Here's how the part is built. I have some questions about the finished solid (model axes, mm). Face numbers are marked on the shaded views. Coordinates: 2 decimals unless noted, no trailing zeros. Write each loop counter-clockwise with the first axis right and the second up, starting at its lowest first coordinate (ties: lowest second). Pieces come first, ordered by that corner, then holes. Notation, with made-up numbers: (-37.75, -6) -> (4.25, -6) arc R12 ccw to (4.25, 5) -> close; hole circle Ø11 at (17, -13). An arc over 180 degrees is marked (long way). Put each result on its own line as item: value.
```python
from build123d import *

# Parameters (mm, degrees)
ESQUISSE1_R                  = 3.4
BOSS_EXTRU_1_DEPTH           = 28
ENL_V_MAT_EXTRU_1_DEPTH      = 29.409857444
ENL_V_MAT_EXTRU_1_DEPTH_BACK = 29.409857444
ESQUISSE2_R                  = 2
CHANFREIN1_SIZE              = 0.5
ESQUISSE3_W                  = 6.25957
ESQUISSE3_H                  = 2.330719663
ENL_V_MAT_EXTRU_2_DEPTH      = 2


with BuildPart() as part:
    # Esquisse1 → Boss.-Extru.1 (new body)
    with BuildSketch(Plane.XY):
        Circle(ESQUISSE1_R)
    extrude(amount=BOSS_EXTRU_1_DEPTH)

    # Esquisse2 → Enlèv. mat.-Extru.1 (cut, two sides: drawn at the far end of the back side and taken through both)
    with BuildSketch(Plane(origin=(0, 0, 0), x_dir=(1, 0, 0), z_dir=(0, 1, 0)).offset(-ENL_V_MAT_EXTRU_1_DEPTH_BACK)):
        with Locations(Location((0, -4.5, 0), (0, 0, 270))):
            Circle(ESQUISSE2_R)
        with Locations(Location((0, -23.5, 0), (0, 0, 270))):
            Circle(ESQUISSE2_R)
    extrude(amount=ENL_V_MAT_EXTRU_1_DEPTH + ENL_V_MAT_EXTRU_1_DEPTH_BACK, mode=Mode.SUBTRACT)

    # Chanfrein1
    chanfrein1_edges = [part.edges().sort_by_distance(p)[0] for p in [
        (-3.4, 0, 0),
        (-3.4, 0, 28),
    ]]
    chamfer(chanfrein1_edges, length=CHANFREIN1_SIZE)

    # Esquisse3 → Enlèv. mat.-Extru.2 (cut)
    with BuildSketch(Plane.XY.offset(28)):
        with Locations((0, 4.365359832)):
            Rectangle(ESQUISSE3_W, ESQUISSE3_H)
        with Locations((0, -4.365359832)):
            Rectangle(ESQUISSE3_W, ESQUISSE3_H)
    extrude(amount=-ENL_V_MAT_EXTRU_2_DEPTH, mode=Mode.SUBTRACT)


solid = part.part
```
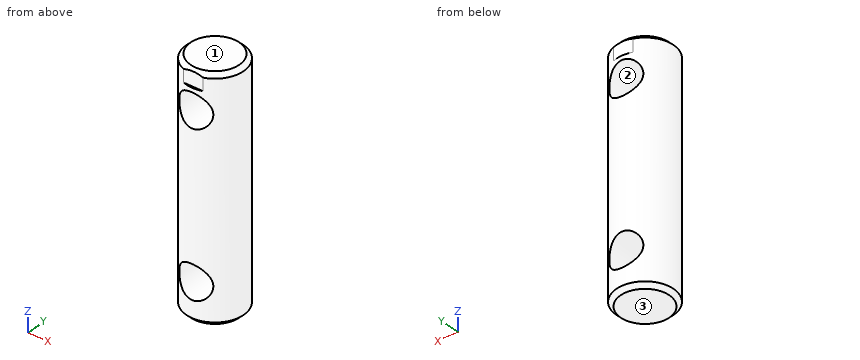
Item 1: Imagine slicing it at D-D on z = 8.25. Write out the boundary of the cut face in (x, y), then the cut area to 3 significant figures.
Output:
outline: circle Ø6.8 at (0, 0)
area: 36.3 mm²
Item 2: For P1, Ø1.4, axis at x = 0, z = 27, coming from the +Y side; P2, Ø4, axis at y = 2.5, z = 19, coming from the +X side, each with a flat end and sliding along its axis, tell me the tip position at first contact or that it passes through.
Output:
P1: stops at y = 3.2
P2: stops at x = 3.36
Item 3: Imagine slicing it at B-B on y = 2. State how many separate pieces and enclosed holes the cut face has, then the cut area to 3 significant figures.
Output:
separate pieces: 1
enclosed holes: 2
area: 128 mm²
Item 4: Please list where these lines run through material, in increasing order: line 1 along Z through (x, y) = (0, 0); line 2 along Z through (x, y) = (-1.5, -0.75); line 3 along X through (y, z) = (1.75, 25.25). Write a range as from..to.
Output:
line 1: z = 0..2.5, 6.5..21.5, 25.5..28
line 2: z = 0..3.18, 5.82..22.18, 24.82..28
line 3: x = -2.92..-0.97, 0.97..2.92
Item 5: If we mould it in two halves opening along Z, with no side actions, what happens to the marked faces 1, 2 and 3? For each: released by +Z, released by -Z, zero draft, split by the parting line, or undercut.
Output:
face 1: released by +Z
face 2: undercut
face 3: released by -Z
Item 6: Imagine slicing it at A-A on z = 24. Write out the boundary of the cut face in (x, y).
Output:
outline: (-1.94, -2.79) -> (-1.94, 2.79) arc R3.4 ccw to start; (1.94, -2.79) arc R3.4 ccw to (1.94, 2.79) -> close
